from build123d import *

# Parameters (mm, degrees)
SKETCH1_R               = 8.5
BOSS_EXTRUDE1_DEPTH     = 29
SKETCH2_W               = 5.55
SKETCH2_H               = 10
CUT_EXTRUDE1_DEPTH      = 10
CUT_EXTRUDE1_DEPTH_BACK = 10


with BuildPart() as part:
    # Sketch1 → Boss-Extrude1 (new body)
    with BuildSketch(Plane(origin=(0, 0, 0), x_dir=(1, 0, 0), z_dir=(0, 1, 0))):
        with Locations(Location((0, 0, 0), (0, 0, 90))):
            Circle(SKETCH1_R)
        with BuildLine():
            ThreePointArc((-5.549518778, 0.143428015), (-5.693479971, 0.065679427), (-5.749324893, -0.08810943))
            ThreePointArc((-5.749324893, -0.08810943), (-5.66264458, -0.998477022), (-5.432733377, -1.883589143))
            ThreePointArc((-5.432733377, -1.883589143), (-5.327657428, -2.009003309), (-5.165786574, -2.032825456))
            ThreePointArc((-5.165786574, -2.032825456), (-4.232699161, -2.44375), (-4.343371773, -3.457289676))
            ThreePointArc((-4.343371773, -3.457289676), (-4.403676616, -3.609385021), (-4.347602736, -3.763090545))
            ThreePointArc((-4.347602736, -3.763090545), (-3.696028756, -4.404755548), (-2.950967451, -4.935006697))
            ThreePointArc((-2.950967451, -4.935006697), (-2.789859933, -4.963538005), (-2.650547084, -4.877738248))
            ThreePointArc((-2.650547084, -4.877738248), (-1.671623451, -4.592747684), (-1.104912844, -5.440303105))
            ThreePointArc((-1.104912844, -5.440303105), (-1.053344031, -5.595578104), (-0.911588941, -5.677279771))
            ThreePointArc((-0.911588941, -5.677279771), (0, -5.75), (0.911588941, -5.677279771))
            ThreePointArc((0.911588941, -5.677279771), (1.053344031, -5.595578104), (1.104912844, -5.440303105))
            ThreePointArc((1.104912844, -5.440303105), (1.671623451, -4.592747684), (2.650547084, -4.877738248))
            ThreePointArc((2.650547084, -4.877738248), (2.789859933, -4.963538005), (2.950967451, -4.935006697))
            ThreePointArc((2.950967451, -4.935006697), (3.696028756, -4.404755548), (4.347602736, -3.763090545))
            ThreePointArc((4.347602736, -3.763090545), (4.403676616, -3.609385021), (4.343371773, -3.457289676))
            ThreePointArc((4.343371773, -3.457289676), (4.232699161, -2.44375), (5.165786574, -2.032825456))
            ThreePointArc((5.165786574, -2.032825456), (5.327657428, -2.009003309), (5.432733377, -1.883589143))
            ThreePointArc((5.432733377, -1.883589143), (5.66264458, -0.998477022), (5.749324893, -0.08810943))
            ThreePointArc((5.749324893, -0.08810943), (5.693479971, 0.065679427), (5.549518778, 0.143428015))
            ThreePointArc((5.549518778, 0.143428015), (4.813247893, 0.848705468), (5.263897115, 1.76326896))
            ThreePointArc((5.263897115, 1.76326896), (5.372584803, 1.885566362), (5.372462977, 2.049180705))
            ThreePointArc((5.372462977, 2.049180705), (4.979646072, 2.875), (4.460874036, 3.628099066))
            ThreePointArc((4.460874036, 3.628099066), (4.319240772, 3.710011742), (4.158984271, 3.677034144))
            ThreePointArc((4.158984271, 3.677034144), (3.141624442, 3.744042216), (2.898971694, 4.734310233))
            ThreePointArc((2.898971694, 4.734310233), (2.903620038, 4.897858577), (2.798357442, 5.023116127))
            ThreePointArc((2.798357442, 5.023116127), (1.966615824, 5.40323257), (1.08513064, 5.646679688))
            ThreePointArc((1.08513064, 5.646679688), (0.923980812, 5.61838833), (0.822414801, 5.490115132))
            ThreePointArc((0.822414801, 5.490115132), (0, 4.8875), (-0.822414801, 5.490115132))
            ThreePointArc((-0.822414801, 5.490115132), (-0.923980812, 5.61838833), (-1.08513064, 5.646679688))
            ThreePointArc((-1.08513064, 5.646679688), (-1.966615824, 5.40323257), (-2.798357442, 5.023116127))
            ThreePointArc((-2.798357442, 5.023116127), (-2.903620038, 4.897858577), (-2.898971694, 4.734310233))
            ThreePointArc((-2.898971694, 4.734310233), (-3.141624442, 3.744042216), (-4.158984271, 3.677034144))
            ThreePointArc((-4.158984271, 3.677034144), (-4.319240772, 3.710011742), (-4.460874036, 3.628099066))
            ThreePointArc((-4.460874036, 3.628099066), (-4.979646072, 2.875), (-5.372462977, 2.049180705))
            ThreePointArc((-5.372462977, 2.049180705), (-5.372584803, 1.885566362), (-5.263897115, 1.76326896))
            ThreePointArc((-5.263897115, 1.76326896), (-4.813247893, 0.848705468), (-5.549518778, 0.143428015))
        make_face(mode=Mode.SUBTRACT)
    extrude(amount=BOSS_EXTRUDE1_DEPTH)

    # Sketch2 → Revolve2 (revolve)
    with BuildSketch(Plane.XY, mode=Mode.PRIVATE) as revolve2_sk:
        with Locations((-5.725, 34)):
            Rectangle(SKETCH2_W, SKETCH2_H)
    revolve(revolve2_sk.sketch.rotate(Axis((0, 0, 0), (0, 1, 0)), 270), axis=Axis((0, 0, 0), (0, 1, 0)))

    # Sketch4 → Cut-Extrude1 (cut, two sides: drawn at the far end of the back side and taken through both)
    with BuildSketch(Plane.XY.offset(-CUT_EXTRUDE1_DEPTH_BACK)):
        with BuildLine():
            Line((-0.95, 37.8), (-0.95, 39))
            Line((-0.95, 39), (0.95, 39))
            Line((0.95, 39), (0.95, 37.8))
            ThreePointArc((0.95, 37.8), (0, 36.85), (-0.95, 37.8))
        make_face()
    extrude(amount=CUT_EXTRUDE1_DEPTH + CUT_EXTRUDE1_DEPTH_BACK, mode=Mode.SUBTRACT)


solid = part.part
Build history of the part. All positions in model axes, mm. A direction names the side the tool comes from. Give positions to 0.01 mm unless a question says otherwise; leave off trailing zeros. Order: outer loops, then holes, each group sorted by start corner. A loop starts at its lowest first (then second) coordinate and runs counter-clockwise, first axis right, second up. Notation, with made-up numbers: M -34.75,-0.5 L 3.25,-0.5 A29 ccw 3.25,20.5 Z; hole C 74.5,-14.5 d11. An arc over 180 degrees is marked long. Put each result on its own line as item: value.
Item 1: Which spindle directions (+Z, -Z, +X, -X, +Y, -Y) get a long thin tool onto all of the face, cutting with end or side? Do faces 4 (the face through (5.66, 14.3, 1.01)), 5 (the face through (-0.95, 38, 6)). Say none if no direction does.
Results are:
face 4: -Y
face 5: +Z, -Z, +Y
Item 2: Cut at A-A on x = 0. Write the cut outline in (y, z), then the cut area to 3 significant figures.
Results are:
outline: M 0,-8.5 L 36.85,-8.5 L 36.85,-2.95 L 29,-2.95 L 29,-4.89 L 0,-4.89 Z; M 0,5.75 L 29,5.75 L 29,2.95 L 36.85,2.95 L 36.85,8.5 L 0,8.5 Z
area: 272 mm2
Item 3: Cut at B-B on z = -1. Write the cut outline in (x, y), then the cut area to 3 significant figures.
Results are:
outline: M -8.44,0 L -4.8,0 L -4.8,29 L -2.78,29 L -2.78,39 L -8.44,39 Z; M 2.78,29 L 4.8,29 L 4.8,0 L 8.44,0 L 8.44,39 L 2.78,39 Z
area: 324 mm2
Item 4: Pull direction Z, two halves, no side cores. Call faces 1 (the face through (1.13, 34.07, -2.725)), 2 (the face through (1.657, 14.297, 4.598)), 3 (the face through (5, 39, 0)): +Z half, -Z half, draft (parallel to the pull), parting line (faces both ways), or undercut.
Results are:
face 1: undercut
face 2: undercut
face 3: draft
Item 5: Drop flat-ended pins along their axis: pin 1 Ø1.3 at (y, z) = (38.5, -5) entering from -X; pin 2 Ø4 at (x, y) = (-3, 30.5) entering from +Z; pin 3 Ø0.6 at (y, z) = (38.5, 5.5) entering from +X. Give the stop position or say it passes through.
Results are:
pin 1: x = -7.3
pin 2: z = 8.44
pin 3: x = 6.72
Item 6: Wall check: probe 1 along X at (y, z) = (36.5, 0); probe 2 along Y at (x, z) = (1.75, -5.25); probe 3 along X at (y, z) = (17, 5.5). Give the ranges that are in metal, low to high.
Results are:
probe 1: -8.5 to -2.95, 2.95 to 8.5
probe 2: 29 to 39
probe 3: -6.48 to -1.1, 1.1 to 6.48
Item 7: Cut at D-D on x = -6.5. Write the cut outline in (y, z), then the cut area to 3 significant figures.
Results are:
outline: M 0,-5.48 L 39,-5.48 L 39,5.48 L 0,5.48 Z
area: 427 mm2
Item 8: Cut at C-C on y = 29.5. Write the cut outline in (x, z).
Results are:
outline: C 0,0 d17; hole C 0,0 d5.9
